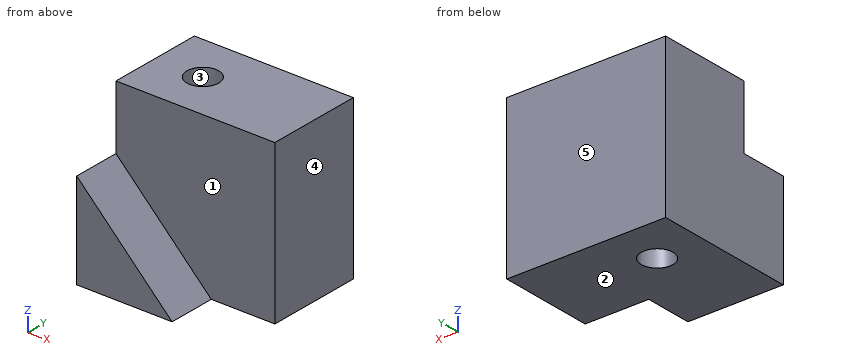
```python
from build123d import *

# Parameters (mm, degrees)
F1_DEPTH = 15
F3_W     = 50
F3_H     = 50
F4_DEPTH = 30
F5_R     = 5
F6_DEPTH = 50


with BuildPart() as f1:
    # F0 (on Front) → F1 (new body)
    with BuildSketch(Plane.XZ):
        Polygon((0, 30), (0, 0), (30, 0), align=None)
    extrude(amount=-F1_DEPTH)

    # F3 (on offset) → F4 (join)
    with BuildSketch(Plane.XZ.offset(-15)):
        with Locations((25, 25)):
            Rectangle(F3_W, F3_H)
    extrude(amount=-F4_DEPTH)

    # F5 (on face) → F6 (cut, through all)
    with BuildSketch(Plane.XY.offset(50)):
        with Locations((15, 30)):
            Circle(F5_R)
    extrude(amount=-F6_DEPTH, mode=Mode.SUBTRACT)


solid = f1.part
```
Verification items for the finished model (mm, model axes). Face numbers are marked on the shaded views. A direction names the side the tool comes from. Give positions to 0.01 mm unless a question says otherwise; leave off trailing zeros. Loops run counter-clockwise (first coordinate to the right, second up) from the corner with the lowest first, then second, coordinate; pieces in that order, holes last.
1. Section check B-B, the plane z = 12.5. Enter the section's corners in (x, y), then the cut area to 3 significant figures.
2. Mould release check, pull along X, two halves, no side actions. Record for the marked faces 3, 4 and 5: released by +X, released by -X, zero draft, split by the parting line, or undercut.
3. Go/stop test with flat-tipped pins: pin 1 Ø12 at (y, z) = (12, 31.5) entering from -X; pin 2 Ø4 at (x, z) = (36.5, 35) entering from -Y. Record where each tip stops, or that it passes through.
4. Section check D-D, the plane y = 11.5. Enter the section's corners in (x, z).
5. Thickness scan on line 1 (Y direction, x = 15, z = 29); line 2 (Y direction, x = 37.5, z = 43.5); line 3 (Y direction, x = 15, z = 4). Record the ranges inside material, lowest first.
6. Section check C-C, the plane x = 15. Enter the section's corners in (y, z), then the cut area to 4 significant figures.
7. Set-up check for the marked faces 1 and 2: record each of +Z, -Z, +X, -X, +Y, -Y from which the full face is reachable in a straight line by a thin tool's end or side.
8. Section check A-A, the plane y = 30. Enter the section's corners in (x, z).
Geometry says:
1. outline: (0, 0) - (17.5, 0) - (17.5, 15) - (50, 15) - (50, 45) - (0, 45) - close; hole circle Ø10 at (15, 30)
1. area: 1,680 mm2
2. face 3: undercut
2. face 4: released by +X
2. face 5: zero draft
3. pin 1: stops at x = 0
3. pin 2: stops at y = 15
4. outline: (0, 0) - (30, 0) - (0, 30) - close
5. line 1: y = 15 to 25, 35 to 45
5. line 2: y = 15 to 45
5. line 3: y = 0 to 25, 35 to 45
6. outline: (0, 0) - (25, 0) - (25, 50) - (15, 50) - (15, 15) - (0, 15) - close; (35, 0) - (45, 0) - (45, 50) - (35, 50) - close
6. area: 1,225 mm2
7. face 1: +Z, +X, -Y
7. face 2: -Z, +X, -X, +Y, -Y
8. outline: (0, 0) - (10, 0) - (10, 50) - (0, 50) - close; (20, 0) - (50, 0) - (50, 50) - (20, 50) - close
